Verification items for the finished model (mm, model axes). Coordinates: 2 decimals unless noted, no trailing zeros. Order: outer loops, then holes, each group sorted by start corner. A loop starts at its lowest first (then second) coordinate and runs counter-clockwise, first axis right, second up.
Q1. Cross-section at A-A, the plane x = -8.5. Record the boundary of the cut face in (y, z), and give its area (3 significant figures).
Q2. Cross-section at C-C, the plane y = -343. Record the boundary of the cut face in (x, z), and give its area (3 significant figures).
Q3. Cross-section at B-B, the plane z = 5.75. Record the boundary of the cut face in (x, y), and give its area (3 significant figures).
Q4. Depth check by flat-ended pin: P1, Ø12, axis at x = -8, z = -8.5, coming from the -Y side. Enter the tip coordinate at first touch or a pass-through.
Q5. Thickness scan on line 1 (X direction, y = 31, z = -6); line 2 (Z direction, x = -20.5, y = 30). Record the ranges inside material, lowest first.
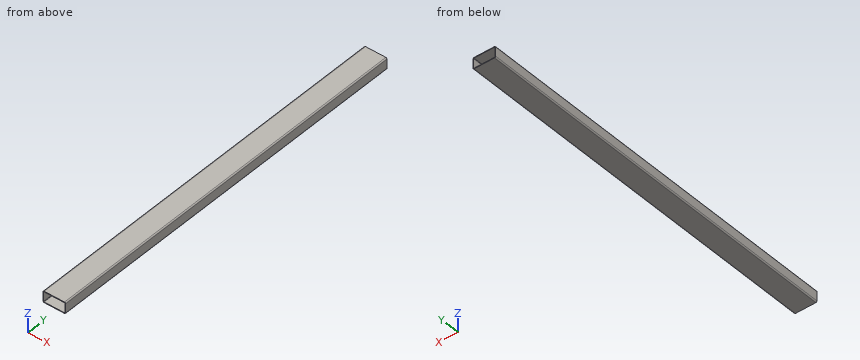
from build123d import *

# Parameters (mm, degrees)
F1_DEPTH = 425


with BuildPart() as f1:
    # F0 (on Front) → F1 (new body, symmetric)
    with BuildSketch(Plane.XZ):
        with BuildLine():
            ThreePointArc((25, 10), (24.267766953, 11.767766953), (22.5, 12.5))
            Line((22.5, 12.5), (-22.5, 12.5))
            ThreePointArc((-22.5, 12.5), (-24.267766953, 11.767766953), (-25, 10))
            Line((-25, 10), (-25, -10))
            ThreePointArc((-25, -10), (-24.267766953, -11.767766953), (-22.5, -12.5))
            Line((-22.5, -12.5), (22.5, -12.5))
            ThreePointArc((22.5, -12.5), (24.267766953, -11.767766953), (25, -10))
            Line((25, -10), (25, 10))
        make_face()
        with BuildLine():
            ThreePointArc((22.5, 11), (23.2071067812, 10.7071067812), (23.5, 10))
            Line((23.5, 10), (23.5, -10))
            ThreePointArc((23.5, -10), (23.2071067812, -10.7071067812), (22.5, -11))
            Line((22.5, -11), (-22.5, -11))
            ThreePointArc((-22.5, -11), (-23.2071067812, -10.7071067812), (-23.5, -10))
            Line((-23.5, -10), (-23.5, 10))
            ThreePointArc((-23.5, 10), (-23.2071067812, 10.7071067812), (-22.5, 11))
            Line((-22.5, 11), (22.5, 11))
        make_face(mode=Mode.SUBTRACT)
    extrude(amount=F1_DEPTH, both=True)


solid = f1.part
Check values:
1. outline: (-425, -12.5) - (425, -12.5) - (425, -11) - (-425, -11) - close; (-425, 11) - (425, 11) - (425, 12.5) - (-425, 12.5) - close
1. area: 2,550 mm2
2. outline: (-25, -10) arc R2.5 ccw to (-22.5, -12.5) - (22.5, -12.5) arc R2.5 ccw to (25, -10) - (25, 10) arc R2.5 ccw to (22.5, 12.5) - (-22.5, 12.5) arc R2.5 ccw to (-25, 10) - close; hole (-23.5, -10) arc R1 ccw to (-22.5, -11) - (22.5, -11) arc R1 ccw to (23.5, -10) - (23.5, 10) arc R1 ccw to (22.5, 11) - (-22.5, 11) arc R1 ccw to (-23.5, 10) - close
2. area: 211 mm2
3. outline: (-25, -425) - (-23.5, -425) - (-23.5, 425) - (-25, 425) - close; (23.5, -425) - (25, -425) - (25, 425) - (23.5, 425) - close
3. area: 2,550 mm2
4. P1: stops at y = -425
5. line 1: x = -25 to -23.5, 23.5 to 25
5. line 2: z = -12.5 to -11, 11 to 12.5
